from build123d import *


with BuildPart() as part:
    # Sketch1 → Revolve1 (revolve)
    with BuildSketch(Plane.XY, mode=Mode.PRIVATE) as revolve1_sk:
        with BuildLine():
            Line((-31.720385191, 56.779614809), (-29.220385191, 56.779614809))
            Line((-29.220385191, 56.779614809), (-22, 64))
            Line((-22, 64), (-16, 64))
            Line((-16, 64), (-16, 56))
            Line((-16, 56), (-19.500883608, 56))
            ThreePointArc((-19.500883608, 56), (-35.117990054, 29.913629212), (-40.555594493, 0))
            Line((-40.555594493, 0), (-50.555594493, 0))
            ThreePointArc((-50.555594493, 0), (-45.723923512, 29.911075571), (-31.720385191, 56.779614809))
        make_face()
    revolve(revolve1_sk.sketch.rotate(Axis((-128.545758478, 0, 0), (1, 0, 0)), 90), axis=Axis((-128.545758478, 0, 0), (1, 0, 0)))


solid = part.part
Check sheet for the modelled part. Datum: model origin and axes. Units: mm. Round coordinates to 2 decimals unless told otherwise and drop trailing zeros. Order: outer loops, then holes, each group sorted by start corner. A loop starts at its lowest first (then second) coordinate and runs counter-clockwise, first axis right, second up.
(1) Scan lines: probe 1 along Y at (x, z) = (-16.75, 0); probe 2 along Z at (x, y) = (-21, 42); probe 3 along Y at (x, z) = (-28, -30.5). Record each from-to range of solid material in increasing order.
(2) Draft check along Y on faces 1 (the flat face through (-16, 57, 0)), 2 (the cylindrical face through (-18.96, 62.48, -13.87)), 3 (the cylindrical face through (-17.77, 49.68, 25.84)). Enter one of: pulls with the +Y half, pulls with the -Y half, needs draft (parallel to the pull), parting line crosses it, or undercut.
(3) Cross-section at A-A, the plane y = 0. Enter the section's corners in (x, z).
(4) Go/stop test with flat-tipped pins: P1, Ø12, axis at x = -29.5, y = -9.5, coming from the -Z side; P2, Ø3, axis at x = -27.5, y = 3.5, coming from the -Z side; P3, Ø3, axis at x = -42, y = -44.5, coming from the +Z side; P4, Ø8, axis at x = -46, z = -4.5, coming from the -Y side. Record where each tip stops, or that it passes through.
(5) Cross-section at C-C, the plane x = -25. Enter the section's corners in (y, z), and give its area (3 significant figures).
Check sheet entries:
1. probe 1: y = -64 to -56, 56 to 64
1. probe 2: z = -48.29 to -34.32, 34.32 to 48.29
1. probe 3: y = -49.33 to -32.35, 32.35 to 49.33
2. face 1: needs draft
2. face 2: parting line crosses it
2. face 3: undercut
3. outline: (-31.72, -56.78) - (-29.22, -56.78) - (-22, -64) - (-16, -64) - (-16, -56) - (-19.5, -56) arc R85 cw to (-19.5, 56) - (-16, 56) - (-16, 64) - (-22, 64) - (-29.22, 56.78) - (-31.72, 56.78) arc R95 ccw to start
4. P1: stops at z = -61.84
4. P2: stops at z = -59.9
4. P3: passes through
4. P4: stops at y = -39.15
5. outline: circle Ø122 at (0, 0); hole circle Ø98.03 at (0, 0)
5. area: 4,140 mm2
